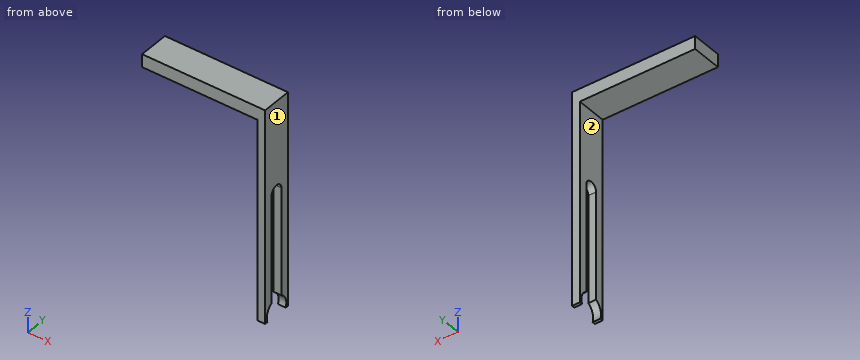
from build123d import *

# Parameters (mm, degrees)
F2_DEPTH = 1.8
F3_W     = 7
F3_H     = 3
F4_DEPTH = 26.8


with BuildPart() as f2:
    # F0 (on Right) → F2 (new body)
    with BuildSketch(Plane.YZ):
        with BuildLine():
            Line((-1.35995, -11.224572), (-1.35995, 13.775428))
            ThreePointArc((-1.35995, 13.775428), (0.14005, 15.275428), (1.64005, 13.775428))
            Line((1.64005, 13.775428), (1.64005, -11.224572))
            ThreePointArc((1.64005, -11.224572), (2.962893, -12.806991), (2.951484, -14.869473))
            Line((2.951484, -14.869473), (3.64005, -14.869473))
            Line((3.64005, -14.869473), (3.64005, 34.775428))
            Line((3.64005, 34.775428), (-3.35995, 34.775428))
            Line((-3.35995, 34.775428), (-3.35995, -14.869473))
            Line((-3.35995, -14.869473), (-2.671383, -14.869473))
            ThreePointArc((-2.671383, -14.869473), (-2.682792, -12.806991), (-1.35995, -11.224572))
        make_face()
    extrude(amount=F2_DEPTH)

    # F3 (on face) → F4 (join)
    with BuildSketch(Plane.YZ):
        with Locations((0.14005, 33.275428)):
            Rectangle(F3_W, F3_H)
    extrude(amount=-F4_DEPTH)


solid = f2.part
The listing builds one solid part. Answer for the finished solid, in the listing's coordinates (mm). Face numbers are marked on the shaded views. A direction names the side the tool comes from. Round coordinates to 2 decimals unless told otherwise and drop trailing zeros. Order: outer loops, then holes, each group sorted by start corner. A loop starts at its lowest first (then second) coordinate and runs counter-clockwise, first axis right, second up. Notation, with made-up numbers: (2, -17) - (45, -17) arc R21 ccw to (45, 15) - close; hole circle Ø5 at (51, -33.75). An arc over 180 degrees is marked (long way). Write item = value, one per line. Start each with the question number.
1) For the marked faces 1 and 2, determine the directions among +Z, -Z, +X, -X, +Y, -Y from which every point of the face is accessible in a straight line to the end or side of a thin tool.
2) Section D-D, the plane z = 22.5 is taken. Write down the section's boundary in (x, y), plus the area to 3 significant figures.
3) Straight lines are drawn through the part: L1, parallel to Z at x = -12, y = -0.5; L2, parallel to X at y = -1.25, z = 31.5; L3, parallel to Y at x = 0.5, z = -0.5. For each, find the intervals that lie inside material, in ascending order.
4) Given pin 1 (1.5 mm diameter, centred on x = -7, y = -2, fed in from -Z); pin 2 (2 mm diameter, centred on y = -1, z = 3.5, fed in from -X), each flat-ended and moving along its own axis, determine where each tip first touches the part or whether it passes through.
5) Section A-A, the plane z = -10.5 is taken. Write down the section's boundary in (x, y).
6) Section B-B, the plane x = -23 is taken. Write down the section's boundary in (y, z).
7) Section C-C, the plane y = 0 is taken. Write down the section's boundary in (x, z).
Results list:
q1.face_1 = +Z, -Z, +X, +Y, -Y
q1.face_2 = -Z, -X, +Y, -Y
q2.outline = (0, -3.36) - (1.8, -3.36) - (1.8, 3.64) - (0, 3.64) - close
q2.area = 12.6 mm^2
q3.L1 = 31.78 to 34.78
q3.L2 = 0 to 1.8
q3.L3 = -3.36 to -1.36, 1.64 to 3.64
q4.pin_1 = 31.78
q4.pin_2 = 0
q5.outline = (0, -3.36) - (1.8, -3.36) - (1.8, -1.36) - (0, -1.36) - close; (0, 1.64) - (1.8, 1.64) - (1.8, 3.64) - (0, 3.64) - close
q6.outline = (-3.36, 31.78) - (3.64, 31.78) - (3.64, 34.78) - (-3.36, 34.78) - close
q7.outline = (-26.8, 31.78) - (0, 31.78) - (0, 15.27) - (1.8, 15.27) - (1.8, 34.78) - (-26.8, 34.78) - close
